Here's how the part is built. I have some questions about the finished solid (model axes, mm). Round coordinates to 2 decimals unless told otherwise and drop trailing zeros. Write each loop counter-clockwise with the first axis right and the second up, starting at its lowest first coordinate (ties: lowest second). Pieces come first, ordered by that corner, then holes. Notation, with made-up numbers: (44.25, 2) - (79.25, 2) arc R22 cw to (79.25, 19) - close; hole circle Ø10 at (-39, -7). An arc over 180 degrees is marked (long way). Write item = value, one per line. Start each with the question number.
Item 1: If we section it at A-A (x = 0): Please give me the cut outline in (y, z).
Item 2: Thinking about a two-plate mould opening in Z: for faces 1 (the face through (-1, 0, 80)), 2 (the face through (29.09, -0.08, 63.94)), 3 (the face through (-1, 6, 39)), which applies, pulls with the +Z half, pulls with the -Z half, needs draft (parallel to the pull), parting line crosses it, or undercut?
Item 3: If we section it at D-D (x = -50.5): Please give me the cut outline in (y, z).
Item 4: If I drill on line 1 along X through (y, z) = (-2.75, 47.5); line 2 along Z through (x, y) = (-30, 1.25) (3 decimals); line 3 along Z through (x, y) = (-17, -5.5), over which ranges is the centre line in solid material (lowest first)? Write a range as [from, to].
Item 5: If we section it at B-B (z = 54.5): Please give me the cut outline in (x, y), and give its area (3 significant figures).
Item 6: For P1, Ø3, axis at x = 15.5, z = 41.5, coming from the -Y side, with a flat end and sliding along its axis, tell me the tip position at first contact or that it passes through.
Item 7: If we section it at C-C (y = 1): Give the number of separate pieces and of enclosed holes in the cut face, and give its area (3 significant figures).
```python
from build123d import *

# Parameters (mm, degrees)
SKETCH_W      = 120
SKETCH_H      = 12
PAD_DEPTH     = 80
SKETCH001_R   = 2.25
SKETCH001_R_2 = 7
SKETCH001_R_3 = 16
SKETCH001_R_4 = 1.75
SKETCH001_R_5 = 2.5
SKETCH001_R_6 = 1
POCKET_DEPTH  = 12.001


with BuildPart() as part:
    # Sketch → Pad (new body)
    with BuildSketch(Plane.XY):
        Rectangle(SKETCH_W, SKETCH_H)
    extrude(amount=PAD_DEPTH)

    # Sketch001 → Pocket (cut, through all)
    with BuildSketch(Plane.XZ.offset(6)):
        with Locations((-49.475, 7.5)):
            Circle(SKETCH001_R)
        with Locations((-32.575, 7.5)):
            Circle(SKETCH001_R)
        with Locations((32.575, 7.5)):
            Circle(SKETCH001_R)
        with Locations((49.475, 7.5)):
            Circle(SKETCH001_R)
        with Locations((-30, 57)):
            Circle(SKETCH001_R_2)
        with Locations((30, 57)):
            Circle(SKETCH001_R_2)
        with Locations((0, 57)):
            Circle(SKETCH001_R_3)
        with Locations((-15.5, 72.5)):
            Circle(SKETCH001_R_4)
        with Locations((-15.5, 41.5)):
            Circle(SKETCH001_R_4)
        with Locations((15.5, 41.5)):
            Circle(SKETCH001_R_4)
        with Locations((15.5, 72.5)):
            Circle(SKETCH001_R_4)
        with Locations((-30, 68.575)):
            Circle(SKETCH001_R_5)
        with Locations((-30, 45.425)):
            Circle(SKETCH001_R_5)
        with Locations((30, 68.575)):
            Circle(SKETCH001_R_5)
        with Locations((30, 45.425)):
            Circle(SKETCH001_R_5)
        with Locations((-55, 54.5)):
            Circle(SKETCH001_R)
        with Locations((55, 54.5)):
            Circle(SKETCH001_R)
        with Locations((-15.5, 31)):
            Circle(SKETCH001_R_6)
        with Locations((15.5, 31)):
            Circle(SKETCH001_R_6)
    extrude(amount=-POCKET_DEPTH, mode=Mode.SUBTRACT)


solid = part.part
```
Reply:
q1.outline = (-6, 0) - (6, 0) - (6, 41) - (-6, 41) - close; (-6, 73) - (6, 73) - (6, 80) - (-6, 80) - close
q2.face_1 = pulls with the +Z half
q2.face_2 = undercut
q2.face_3 = needs draft
q3.outline = (-6, 0) - (6, 0) - (6, 5.5) - (-6, 5.5) - close; (-6, 9.5) - (6, 9.5) - (6, 80) - (-6, 80) - close
q4.line_1 = [-60, -31.39], [-28.61, -12.87], [12.87, 28.61], [31.39, 60]
q4.line_2 = [0, 42.925], [47.925, 50], [64, 66.075], [71.075, 80]
q4.line_3 = [0, 40.6], [42.4, 71.6], [73.4, 80]
q5.outline = (-60, -6) - (-57.25, -6) - (-57.25, 6) - (-60, 6) - close; (-52.75, -6) - (-36.54, -6) - (-36.54, 6) - (-52.75, 6) - close; (-23.46, -6) - (-15.8, -6) - (-15.8, 6) - (-23.46, 6) - close; (15.8, -6) - (23.46, -6) - (23.46, 6) - (15.8, 6) - close; (36.54, -6) - (52.75, -6) - (52.75, 6) - (36.54, 6) - close; (57.25, -6) - (60, -6) - (60, 6) - (57.25, 6) - close
q5.area = 639 mm2
q6.P1 = through
q7.separate_pieces = 1
q7.enclosed_holes = 19
q7.area = 8,270 mm2
